```python
from build123d import *

# Parameters (mm, degrees)
COPYSKETCH001_R    = 18
PAD_DEPTH          = 15
PAD001_DEPTH       = 15
POLARPATTERN_COUNT = 24
SKETCH_R           = 1.25
POCKET_DEPTH       = 15


with BuildPart() as part:
    # CopySketch001 → Pad (new body)
    with BuildSketch(Plane.XY):
        Circle(COPYSKETCH001_R)
    extrude(amount=PAD_DEPTH)

    # Sketch001 (on Face3 of Pad) → Pad001 (join)
    with BuildSketch(Plane.XY.offset(15)):
        with BuildLine():
            ThreePointArc((16.375899, 38.346054), (7.775164, 28.601805), (1.916739, 17))
            Line((-1.083261, 17), (1.916739, 17))
            ThreePointArc((14.505004, 40.479684), (5.147213, 29.777962), (-1.083261, 17))
            Line((14.505004, 40.479684), (16.375899, 38.346054))
        make_face()
    pad001 = extrude(amount=-PAD001_DEPTH)

    # PolarPattern: Pad001 ×24 about axis
    polarpattern_axis = Axis((0, 0, 0), (0, 0, 1))
    for i in range(1, POLARPATTERN_COUNT):
        add(pad001.rotate(polarpattern_axis, i * 360 / POLARPATTERN_COUNT))

    # Sketch (on Face57 of PolarPattern) → Pocket (cut)
    with BuildSketch(Plane.XY.offset(15)):
        with Locations((0, 15)):
            Circle(SKETCH_R)
        with Locations((-15, 0)):
            Circle(SKETCH_R)
        with Locations((0, -15)):
            Circle(SKETCH_R)
        with Locations((15, 0)):
            Circle(SKETCH_R)
    extrude(amount=-POCKET_DEPTH, mode=Mode.SUBTRACT)


solid = part.part
```
The listing builds one solid part. Answer for the finished solid, in the listing's coordinates (mm). A direction names the side the tool comes from. Give positions to 0.01 mm unless a question says otherwise; leave off trailing zeros. Order: outer loops, then holes, each group sorted by start corner. A loop starts at its lowest first (then second) coordinate and runs counter-clockwise, first axis right, second up.
Item 1: For a pull along X with two mould halves and no side action, classify faces 6 (the face through (41.86, 6.35, 7.6)), 7 (the face through (-10.382, 29.073, 7.605)), 8 (the face through (10.382, -29.073, 7.605)), 9 (the face through (-42.077, 4.697, 7.605)) as pulls with the +X half, pulls with the -X half, needs draft (parallel to the pull), parting line crosses it, or undercut.
From the geometry:
face 6: pulls with the +X half
face 7: undercut
face 8: undercut
face 9: pulls with the -X half
Item 2: The part is cut by section A-A, the plane x = 31. Give the vertices of the cut face in (y, z).
From the geometry:
outline: (-22.41, 0) - (-17.19, 0) - (-17.19, 15) - (-22.41, 15) - close; (-9.5, 0) - (-5.98, 0) - (-5.98, 15) - (-9.5, 15) - close; (-0.6, 0) - (2.42, 0) - (2.42, 15) - (-0.6, 15) - close; (7.34, 0) - (10.2, 0) - (10.2, 15) - (7.34, 15) - close; (15.46, 0) - (18.31, 0) - (18.31, 15) - (15.46, 15) - close; (24.49, 0) - (27.41, 0) - (27.41, 15) - (24.49, 15) - close
Item 3: The part is cut by section C-C, the plane x = -23.5. Count the separate pieces of the cut face and the enclosed holes in it, and give its area (3 significant figures).
From the geometry:
separate pieces: 8
enclosed holes: 0
area: 445 mm2
Item 4: Find the intervals of material crossed by probe 1 along Y at (x, z) = (-30, 11.5); probe 2 along X at (y, z) = (30.5, 10.25); probe 3 along Y at (x, z) = (34.5, 11.25), in increasing order.
From the geometry:
probe 1: y = -27.17 to -24.23, -18.22 to -15.36, -10.3 to -7.45, -2.77 to 0.23, 5.3 to 8.76, 15.82 to 20.78
probe 2: x = -27.29 to -24.37, -18.26 to -15.41, -10.25 to -7.4, -2.6 to 0.41, 5.64 to 9.13, 16.49 to 21.58
probe 3: y = -24.9 to -22.84, -12.44 to -8.67, -2.08 to 1.04, 6.81 to 9.69, 15.64 to 18.48
Item 5: The part is cut by section B-B, the plane y = -37. Give the vertices of the cut face in (x, z), and give its area (3 significant figures).
From the geometry:
outline: (-14.9, 0) - (-10.89, 0) - (-10.89, 15) - (-14.9, 15) - close; (-3.33, 0) - (-0.13, 0) - (-0.13, 15) - (-3.33, 15) - close; (6.27, 0) - (9.18, 0) - (9.18, 15) - (6.27, 15) - close; (15.62, 0) - (18.46, 0) - (18.46, 15) - (15.62, 15) - close
area: 194 mm2
Item 6: Given pin 1 Ø12 at (x, y) = (-28.5, -20.5) entering from -Z; pin 2 Ø4 at (y, z) = (23, 8.5) entering from -X; pin 3 Ø4 at (x, z) = (9, 4.5) entering from +Y; pin 4 Ø8 at (x, z) = (19, 10.5) entering from -Y, each flat-ended and moving along its own axis, determine where each tip first touches the part or whether it passes through.
From the geometry:
pin 1: stops at z = 0
pin 2: stops at x = -35.35
pin 3: stops at y = 37.11
pin 4: stops at y = -38.88
Item 7: Which of the six approach directions +Z, -Z, +X, -X, +Y, -Y give full straight-line access (tool end or side, diameter ignored) to faces 1 (the face through (17.553, -25.395, 7.605)), 2 (the face through (6.35, -41.86, 7.6)), 3 (the face through (38.79, 16.97, 7.6)), 4 (the face through (-4.697, -42.077, 7.605)), 5 (the face through (-39.428, 15.427, 7.605))?
From the geometry:
face 1: +Z, -Z
face 2: +Z, -Z, -Y
face 3: +Z, -Z, +X
face 4: +Z, -Z, -X, -Y
face 5: +Z, -Z, -X, +Y
